Here's how the part is built. I have some questions about the finished solid (model axes, mm). Face numbers are marked on the shaded views. A direction names the side the tool comes from. Give positions to 0.01 mm unless a question says otherwise; leave off trailing zeros. Order: outer loops, then holes, each group sorted by start corner. A loop starts at its lowest first (then second) coordinate and runs counter-clockwise, first axis right, second up. Notation, with made-up numbers: M 88,67 L 145,67 A27 ccw 145,104 Z; hole C -21.5,-32.75 d11. An arc over 180 degrees is marked long. Use one line per item in the form item = value.
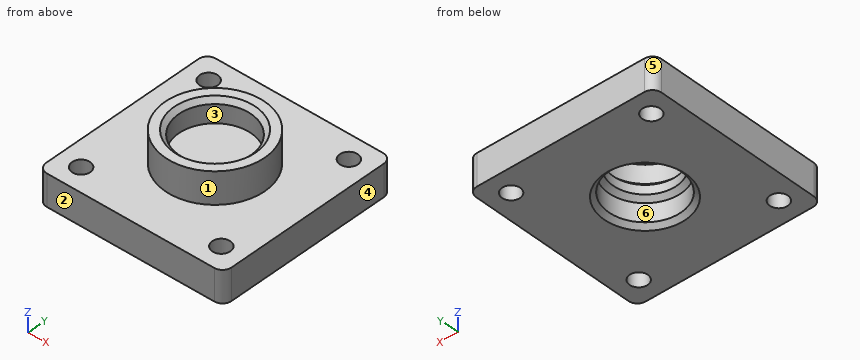
Autodesk Inventor part; units mm, degrees
ref_plane "Work Plane1" through (0, 0, 7) normal (0, 0, -1) x (-1, 0, 0)
ref_plane "YZ Plane" through (0, 0, 0) normal (1, 0, 0) x (0, 1, 0)
ref_plane "XZ Plane" through (0, 0, 0) normal (0, 1, 0) x (-1, 0, 0)
sketch "Sketch1" plane through (0, 0, 0) normal (0, 0, 1) x (1, 0, 0)
  line L0 (5, 36) -> (36, 36) construction
  line L1 (36, 36) -> (36, 5) construction
  line L2 (36, 5) -> (5, 5) construction
  line L3 (5, 5) -> (5, 36) construction
  line L4 (41, 41) -> (0, 41)
  line L5 (0, 41) -> (0, 0)
  line L6 (0, 0) -> (41, 0)
  line L7 (41, 0) -> (41, 41)
  dimension "d0" = 31
  dimension "d1" = 5
extrude "Extrusion1" add sketch "Sketch1" along normal blind 7
hole "Hole1" at (5, 36, 0) at (36, 36, 0) at (36, 5, 0) at (5, 5, 0) direction (0, 0, 1) diameter 4 end through all
sketch "Sketch2" plane through (0, 0, 7) normal (0, 0, 1) x (1, 0, 0)
  circle A0 centre (20.5, 20.5) radius 11
  circle A1 centre (20.5, 20.5) radius 8 construction
  line L0 (41, 0) -> (41, 41)
  line L1 (41, 41) -> (0, 41)
  point P0 (0, 0)
  point P1 (41, 20.5)
  point P2 (20.5, 41)
  dimension "d11" = 22
  dimension "d12" = 16
extrude "Extrusion2" add sketch "Sketch2" along normal blind 7
sketch "Sketch3" plane through (20.5, 20.5, 14) normal (0, 0, 1) x (1, 0, 0)
  circle A0 centre (0, 0) radius 11
  circle A1 centre (0, 0) radius 8
  point P0 (-20.5, -20.5)
  dimension "d15" = 16
extrude "Extrusion3" cut sketch "Sketch3" against normal through all contours A1
ref_plane "Work Plane1" through (0, 0, 7) normal (0, 0, -1) x (-1, 0, 0)
sketch "Sketch4" plane through (0, 0, 7) normal (0, 0, -1) x (-1, 0, 0)
  circle A0 centre (-20.5, 20.5) radius 8
  circle A1 centre (-20.5, 20.5) radius 11
  circle A2 centre (-20.5, 20.5) radius 7
  point P0 (0, 0)
  dimension "d18" = 1
extrude "Extrusion4" add sketch "Sketch4" along normal mid plane 4 contours A0
chamfer "Chamfer1" distance 1 angle 45 2 edges at (27.5, 20.5, 9) (27.5, 20.5, 5)
fillet "Fillet1" radius 2 4 edges at (0, 41, 3.5) (0, 0, 3.5) (41, 0, 3.5) (41, 41, 3.5)
chamfer "Chamfer2" distance 1 angle 45 2 edges at (12.5, 20.5, 0) (12.5, 20.5, 14)
properties part number "Motor to Bearing Adapter"
Q1. I need wall thicknesses on L1, parallel to X at y = 5, z = 3.25; L2, parallel to Y at x = 20.5, z = 3.7. Which ranges of each line are inside material? Lowest first, please.
Found:
L1 = 0 to 3, 7 to 34, 38 to 41
L2 = 0 to 12.5, 28.5 to 41
Q2. I want a section at C-C on y = 36. Write out the boundary of the cut face in (x, z), then the cut area to 3 significant figures.
Found:
outline = M 0,0 L 3,0 L 3,7 L 0,7 Z; M 7,0 L 34,0 L 34,7 L 7,7 Z; M 38,0 L 41,0 L 41,7 L 38,7 Z
area = 231 mm²
Q3. I want a section at B-B on z = 2.25. Write out the boundary of the cut face in (x, y), then the cut area to 3 significant figures.
Found:
outline = M 0,2 A2 ccw 2,0 L 39,0 A2 ccw 41,2 L 41,39 A2 ccw 39,41 L 2,41 A2 ccw 0,39 Z; hole C 5,5 d4; hole C 5,36 d4; hole C 20.5,20.5 d16; hole C 36,5 d4; hole C 36,36 d4
area = 1,430 mm²
Q4. I'm going to push flat-ended pins straight in: pin 1 Ø4 at (x, y) = (8, 32) entering from -Z; pin 2 Ø6.5 at (x, y) = (36, 36) entering from +Z. Where does each tip first touch, or does it pass through?
Found:
pin_1 = 0
pin_2 = 7
Q5. On a 3-axis mill with a long thin cutter (end or side, diameter ignored), from which of +Z, -Z, +X, -X, +Y, -Y can I reach the whole of each face in a straight line? I mean the marked faces 1 and 2. Say none if no direction works.
Found:
face_1 = +Z
face_2 = +Z, -Z, +X, -X, -Y
Q6. Thinking about a two-plate mould opening in X: for the marked faces 3, 4, 5 and 6, which applies, +X half, -X half, draft (parallel to the pull), parting line (faces both ways), or undercut?
Found:
face_3 = undercut
face_4 = +X half
face_5 = -X half
face_6 = undercut
